from build123d import *

# Parameters (mm, degrees)
SKETCH1_W          = 5.563387429
SKETCH1_H          = 13.5
SKETCH1_W_2        = 6.5
SKETCH1_H_2        = 12.5
FILLET1_R          = 1
SKETCH2_R          = 11.704122172
SKETCH2_R_2        = 1.05
CUT_EXTRUDE1_DEPTH = 1
SKETCH2_3_R        = 1.05
CUT_EXTRUDE2_DEPTH = 38.339657272
SKETCH3_R          = 21.771584826
SKETCH3_R_2        = 12.5
CUT_EXTRUDE3_DEPTH = 1
SKETCH4_R          = 21.771584826
SKETCH4_R_2        = 12.5
CUT_EXTRUDE4_DEPTH = 1


with BuildPart() as part:
    # Sketch1 → Revolve1 (revolve)
    with BuildSketch(Plane(origin=(0, 0, 0), x_dir=(1, 0, 0), z_dir=(0, 1, 0))):
        with Locations((2.781693715, 19.25)):
            Rectangle(SKETCH1_W, SKETCH1_H)
        with Locations((3.25, 6.25)):
            Rectangle(SKETCH1_W_2, SKETCH1_H_2)
    revolve(axis=Axis((6.5, 0, 0), (-1, 0, 0)))

    # Fillet1
    fillet1_edges = [part.edges().sort_by_distance(p)[0] for p in [
        (0, 0, 26),
        (5.563387429, 0, 26),
    ]]
    fillet(fillet1_edges, radius=FILLET1_R)

    # Sketch2 → Cut-Extrude1 (cut)
    with BuildSketch(Plane(origin=(6.5, 0, 0), x_dir=(0, 0, -1), z_dir=(1, 0, 0))):
        Circle(SKETCH2_R)
        with BuildLine():
            Line((6.215873313, -3.090198068), (4.862176877, -0.745527062))
            ThreePointArc((4.862176877, -0.745527062), (3.478259233, -3.478259233), (0.745527062, -4.862176877))
            Line((0.745527062, -4.862176877), (3.090198068, -6.215873313))
            Line((3.090198068, -6.215873313), (3.090198068, -9.784126687))
            Line((3.090198068, -9.784126687), (0, -11.568253373))
            Line((0, -11.568253373), (-3.090198068, -9.784126687))
            Line((-3.090198068, -9.784126687), (-3.090198068, -6.215873313))
            Line((-3.090198068, -6.215873313), (-0.745527062, -4.862176877))
            ThreePointArc((-0.745527062, -4.862176877), (-3.478259233, -3.478259233), (-4.862176877, -0.745527062))
            Line((-4.862176877, -0.745527062), (-6.215873313, -3.090198068))
            Line((-6.215873313, -3.090198068), (-9.784126687, -3.090198068))
            Line((-9.784126687, -3.090198068), (-11.568253373, 0))
            Line((-11.568253373, 0), (-9.784126687, 3.090198068))
            Line((-9.784126687, 3.090198068), (-6.215873313, 3.090198068))
            Line((-6.215873313, 3.090198068), (-4.862176877, 0.745527062))
            ThreePointArc((-4.862176877, 0.745527062), (-3.478259233, 3.478259233), (-0.745527062, 4.862176877))
            Line((-0.745527062, 4.862176877), (-3.090198068, 6.215873313))
            Line((-3.090198068, 6.215873313), (-3.090198068, 9.784126687))
            Line((-3.090198068, 9.784126687), (0, 11.568253373))
            Line((0, 11.568253373), (3.090198068, 9.784126687))
            Line((3.090198068, 9.784126687), (3.090198068, 6.215873313))
            Line((3.090198068, 6.215873313), (0.745527062, 4.862176877))
            ThreePointArc((0.745527062, 4.862176877), (3.478259233, 3.478259233), (4.862176877, 0.745527062))
            Line((4.862176877, 0.745527062), (6.215873313, 3.090198068))
            Line((6.215873313, 3.090198068), (9.784126687, 3.090198068))
            Line((9.784126687, 3.090198068), (11.568253373, 0))
            Line((11.568253373, 0), (9.784126687, -3.090198068))
            Line((9.784126687, -3.090198068), (6.215873313, -3.090198068))
        make_face(mode=Mode.SUBTRACT)
        Polygon((-2.237316109, 6.708284942), (0, 5.416569884), (2.237316109, 6.708284942), (2.237316109, 9.291715058), (0, 10.583430116), (-2.237316109, 9.291715058), align=None)
        with Locations((0, 8)):
            Circle(SKETCH2_R_2, mode=Mode.SUBTRACT)
        Polygon((-6.708284942, -2.237316109), (-5.416569884, 0), (-6.708284942, 2.237316109), (-9.291715058, 2.237316109), (-10.583430116, 0), (-9.291715058, -2.237316109), align=None)
        with Locations((-8, 0)):
            Circle(SKETCH2_R_2, mode=Mode.SUBTRACT)
        Polygon((6.708284942, 2.237316109), (5.416569884, 0), (6.708284942, -2.237316109), (9.291715058, -2.237316109), (10.583430116, 0), (9.291715058, 2.237316109), align=None)
        with Locations((8, 0)):
            Circle(SKETCH2_R_2, mode=Mode.SUBTRACT)
        Polygon((2.237316109, -6.708284942), (0, -5.416569884), (-2.237316109, -6.708284942), (-2.237316109, -9.291715058), (0, -10.583430116), (2.237316109, -9.291715058), align=None)
        with Locations((0, -8)):
            Circle(SKETCH2_R_2, mode=Mode.SUBTRACT)
    extrude(amount=-CUT_EXTRUDE1_DEPTH, mode=Mode.SUBTRACT)

    # Sketch2_3 → Cut-Extrude2 (cut, through all)
    with BuildSketch(Plane(origin=(6.5, 0, 0), x_dir=(0, 0, -1), z_dir=(1, 0, 0))):
        with Locations((0, 8)):
            Circle(SKETCH2_3_R)
        with Locations((8, 0)):
            Circle(SKETCH2_3_R)
        with Locations((0, -8)):
            Circle(SKETCH2_3_R)
        with Locations((-8, 0)):
            Circle(SKETCH2_3_R)
        with BuildLine():
            Line((4.862176877, -0.745527062), (4.431746627, 0))
            Line((4.431746627, 0), (4.862176877, 0.745527062))
            ThreePointArc((4.862176877, 0.745527062), (3.478259233, 3.478259233), (0.745527062, 4.862176877))
            Line((0.745527062, 4.862176877), (0, 4.431746627))
            Line((0, 4.431746627), (-0.745527062, 4.862176877))
            ThreePointArc((-0.745527062, 4.862176877), (-3.478259233, 3.478259233), (-4.862176877, 0.745527062))
            Line((-4.862176877, 0.745527062), (-4.431746627, 0))
            Line((-4.431746627, 0), (-4.862176877, -0.745527062))
            ThreePointArc((-4.862176877, -0.745527062), (-3.478259233, -3.478259233), (-0.745527062, -4.862176877))
            Line((-0.745527062, -4.862176877), (0, -4.431746627))
            Line((0, -4.431746627), (0.745527062, -4.862176877))
            ThreePointArc((0.745527062, -4.862176877), (3.478259233, -3.478259233), (4.862176877, -0.745527062))
        make_face()
        with BuildLine():
            ThreePointArc((-0.745527062, -4.862176877), (0, -4.91900138), (0.745527062, -4.862176877))
            Line((0.745527062, -4.862176877), (0, -4.431746627))
            Line((0, -4.431746627), (-0.745527062, -4.862176877))
        make_face()
        with BuildLine():
            ThreePointArc((-4.862176877, 0.745527062), (-4.91900138, 0), (-4.862176877, -0.745527062))
            Line((-4.862176877, -0.745527062), (-4.431746627, 0))
            Line((-4.431746627, 0), (-4.862176877, 0.745527062))
        make_face()
        with BuildLine():
            Line((0, 4.431746627), (0.745527062, 4.862176877))
            ThreePointArc((0.745527062, 4.862176877), (0, 4.91900138), (-0.745527062, 4.862176877))
            Line((-0.745527062, 4.862176877), (0, 4.431746627))
        make_face()
        with BuildLine():
            Line((4.862176877, 0.745527062), (4.431746627, 0))
            Line((4.431746627, 0), (4.862176877, -0.745527062))
            ThreePointArc((4.862176877, -0.745527062), (4.904774681, -0.373844762), (4.91900138, 0))
            ThreePointArc((4.91900138, 0), (4.904774681, 0.373844762), (4.862176877, 0.745527062))
        make_face()
    extrude(amount=-CUT_EXTRUDE2_DEPTH, mode=Mode.SUBTRACT)

    # Sketch3 → Cut-Extrude3 (cut)
    with BuildSketch(Plane.ZY):
        Circle(SKETCH3_R)
        with Locations(Location((0, 0, 0), (0, 0, 180))):
            Circle(SKETCH3_R_2, mode=Mode.SUBTRACT)
    extrude(amount=-CUT_EXTRUDE3_DEPTH, mode=Mode.SUBTRACT)

    # Sketch4 → Cut-Extrude4 (cut)
    with BuildSketch(Plane(origin=(5.563387429, 0, 0), x_dir=(0, 0, -1), z_dir=(1, 0, 0))):
        with Locations(Location((0, 0, 0), (0, 0, 180))):
            Circle(SKETCH4_R)
        Circle(SKETCH4_R_2, mode=Mode.SUBTRACT)
    extrude(amount=-CUT_EXTRUDE4_DEPTH, mode=Mode.SUBTRACT)


solid = part.part
The listing builds one solid part. Answer for the finished solid, in the listing's coordinates (mm). A direction names the side the tool comes from. Give positions to 0.01 mm unless a question says otherwise; leave off trailing zeros. Write each loop counter-clockwise with the first axis right and the second up, starting at its lowest first coordinate (ties: lowest second). Pieces come first, ordered by that corner, then holes.
1) Section A-A (x = 3.75) is taken. Write down the section's boundary in (y, z).
2) Given P1, Ø1.9, axis at y = -8, z = 0, coming from the +X side; P2, Ø0.5, axis at x = 6, z = 7.5, coming from the -Y side; P3, Ø1.5, axis at y = 14, z = -13, coming from the -X side; P4, Ø0.8, axis at x = 6, y = 9, coming from the -Z side, each flat-ended and moving along its own axis, determine where each tip first touches the part or whether it passes through.
3) A tool of negligible diameter and unlimited length cuts with its end or side. For faces 1 (the face through (2.79, 8.89, -0.56)), 2 (the face through (6.01, -6.07, -1.13)), from which of +Z, -Z, +X, -X, +Y, -Y can it reach the whole face along a straight path? Write none if from no direction.
4) Find the intervals of material crossed by L1, parallel to Y at x = 3.2, z = 0; L2, parallel to Z at x = 5, y = -11; L3, parallel to X at y = 3.5, z = -17, in increasing order.
Response:
1. outline: circle Ø52 at (0, 0); hole circle Ø2.1 at (-8, 0); hole circle Ø9.84 at (0, 0); hole circle Ø2.1 at (0, -8); hole circle Ø2.1 at (0, 8); hole circle Ø2.1 at (8, 0)
2. P1: passes through
2. P2: stops at y = -10.18
2. P3: stops at x = 1
2. P4: stops at z = -9.07
3. face 1: +X, -X
3. face 2: +X
4. L1: y = -26 to -9.05, -6.95 to -4.92, 4.92 to 6.95, 9.05 to 26
4. L2: z = -23.45 to -18.79, -5.94 to 5.94, 18.79 to 23.45
4. L3: x = 1 to 4.56
